Work out the finished part from the listing and answer in its coordinate system (mm). Coordinates: 2 decimals unless noted, no trailing zeros. Order: outer loops, then holes, each group sorted by start corner. A loop starts at its lowest first (then second) coordinate and runs counter-clockwise, first axis right, second up.
1. The part is cut by section B-B, the plane y = 17.5. Give the vertices of the cut face in (x, z), then the cut area to 3 significant figures.
2. The part is cut by section D-D, the plane x = -1.5. Give the vertices of the cut face in (y, z).
3. The part is cut by section A-A, the plane x = 0. Give the vertices of the cut face in (y, z), then the cut area to 3 significant figures.
4. The part is cut by section C-C, the plane z = 3.05. Give the vertices of the cut face in (x, y).
5. Flat-ended cylindrical pins translate along their axes: pin 1 Ø2 at (y, z) = (10, 1.5) entering from -X; pin 2 Ø0.6 at (y, z) = (17.5, 3.5) entering from -X; pin 3 Ø1 at (y, z) = (20.5, 3) entering from -X. Find the tip coordinate at first contact, or state that the pin passes through.
6. Determine the mould class of faces 1 (the flat face through (0, 15, 0)), 2 (the flat face through (0, 30, 2)), 3 (the cylindrical face through (-0.65, 20.07, 2.03)), 4 (the flat face through (0, 0, 2)) for opening direction Y: +Y half, -Y half, draft (parallel to the pull), parting line (faces both ways), or undercut.
7. Find the intervals of material crossed by probe 1 along Y at (x, z) = (0, 2.1); probe 2 along Y at (x, z) = (2.25, 1); probe 3 along X at (y, z) = (23, 1.3), in increasing order.
```python
from build123d import *

# Parameters (mm, degrees)
EXTRUDE_1_DEPTH     = 30
FILLET_1_R          = 0.5
SKETCH_2_R          = 3
CUT_EXTRUDE_1_DEPTH = 30


with BuildPart() as part:
    # Эскиз1 → Бобышка-Вытянуть1 (new body)
    with BuildSketch(Plane(origin=(0, 0, 0), x_dir=(1, 0, 0), z_dir=(0, 1, 0))):
        Polygon((-5, 0), (5, 0), (5, -1.5), (3.5, -2.5), (3.5, -4), (-3.5, -4), (-3.5, -2.5), (-5, -1.5), align=None)
    extrude(amount=EXTRUDE_1_DEPTH)

    # Скругление1
    fillet_1_edges = [part.edges().sort_by_distance(p)[0] for p in [
        (5, 15, 1.5),
        (3.5, 15, 2.5),
        (3.5, 15, 4),
        (-3.5, 15, 4),
        (-3.5, 15, 2.5),
        (-5, 15, 1.5),
    ]]
    fillet(fillet_1_edges, radius=FILLET_1_R)

    # Эскиз2 → Вырез-Вытянуть1 (cut)
    with BuildSketch(Plane.XY.offset(4)):
        with Locations((0, 23)):
            Circle(SKETCH_2_R)
        with Locations((0, 7)):
            Circle(SKETCH_2_R)
    extrude(amount=-CUT_EXTRUDE_1_DEPTH, mode=Mode.SUBTRACT)


solid = part.part
```
Geometry says:
1. outline: (-5, 0) - (5, 0) - (5, 1.23) arc R0.5 ccw to (4.78, 1.65) - (3.72, 2.35) arc R0.5 cw to (3.5, 2.77) - (3.5, 3.5) arc R0.5 ccw to (3, 4) - (-3, 4) arc R0.5 ccw to (-3.5, 3.5) - (-3.5, 2.77) arc R0.5 cw to (-3.72, 2.35) - (-4.78, 1.65) arc R0.5 ccw to (-5, 1.23) - close
1. area: 33.9 mm2
2. outline: (0, 0) - (4.4, 0) - (4.4, 4) - (0, 4) - close; (9.6, 0) - (20.4, 0) - (20.4, 4) - (9.6, 4) - close; (25.6, 0) - (30, 0) - (30, 4) - (25.6, 4) - close
3. outline: (0, 0) - (4, 0) - (4, 4) - (0, 4) - close; (10, 0) - (20, 0) - (20, 4) - (10, 4) - close; (26, 0) - (30, 0) - (30, 4) - (26, 4) - close
3. area: 72.0 mm2
4. outline: (-3.5, 0) - (3.5, 0) - (3.5, 30) - (-3.5, 30) - close; hole circle Ø6 at (0, 7); hole circle Ø6 at (0, 23)
5. pin 1: stops at x = -5
5. pin 2: stops at x = -3.5
5. pin 3: stops at x = -3.58
6. face 1: draft
6. face 2: +Y half
6. face 3: undercut
6. face 4: -Y half
7. probe 1: y = 0 to 4, 10 to 20, 26 to 30
7. probe 2: y = 0 to 5.02, 8.98 to 21.02, 24.98 to 30
7. probe 3: x = -5 to -3, 3 to 5
